Autodesk Inventor part; units mm, degrees
ref_plane "YZ Plane" through (0, 0, 0) normal (1, 0, 0) x (0, 1, 0)
ref_plane "XZ Plane" through (0, 0, 0) normal (0, 1, 0) x (-1, 0, 0)
ref_plane "XY Plane" through (0, 0, 0) normal (0, 0, 1) x (1, 0, 0)
sketch "Sketch1" plane through (0, 0, 0) normal (0, 0, 1) x (1, 0, 0)
  line L0 (0, 0) -> (-25.4, 0)
  line L1 (-25.4, 0) -> (-25.4, 50.8)
  line L2 (-25.4, 50.8) -> (0, 50.8)
  line L3 (0, 50.8) -> (0, 0)
  line L4 (-22.225, 3.175) -> (-3.175, 3.175)
  line L5 (-3.175, 3.175) -> (-3.175, 47.625)
  line L6 (-3.175, 47.625) -> (-22.225, 47.625)
  line L7 (-22.225, 47.625) -> (-22.225, 3.175)
  dimension "d0" = 25.4
  dimension "d1" = 50.8
  dimension "d2" = 3.175
extrude "Extrusion1" add sketch "Sketch1" along normal blind 177.8
sketch "Sketch2" plane through (0, 0, 0) normal (1, 0, 0) x (0, 0, -1)
  circle A0 centre (-152.4, 19.05) radius 14.2875
  circle A1 centre (-25.4, 19.05) radius 14.2875
  circle A2 centre (-88.9, 19.05) radius 14.2875
  line L0 (-177.8, 0) -> (-177.8, 50.8)
  line L1 (0, 50.8) -> (0, 0)
  line L2 (0, 50.8) -> (-177.8, 50.8)
  line L3 (0, 0) -> (-177.8, 0)
  dimension "d5" = 28.575
  dimension "d6" = 28.575
  dimension "d7" = 28.575
  dimension "d8" = 25.4
  dimension "d9" = 25.4
  dimension "d10" = 31.75
  dimension "d11" = 31.75
  dimension "d12" = 19.05
  dimension "a" = 63.5
  dimension "d14" = 63.5
extrude "Extrusion2" cut sketch "Sketch2" against normal blind 209.3722 contours A0 | A1 | A2
properties part number "Clamp Arms"
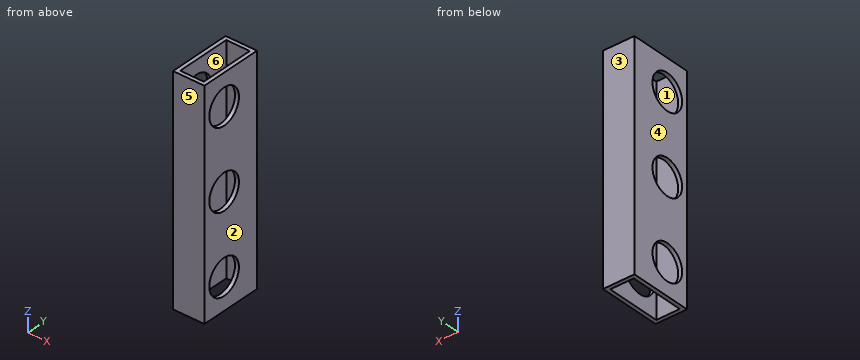
Verification items for the finished model (mm, model axes). Face numbers are marked on the shaded views. A direction names the side the tool comes from. Coordinates: 2 decimals unless noted, no trailing zeros. Order: outer loops, then holes, each group sorted by start corner. A loop starts at its lowest first (then second) coordinate and runs counter-clockwise, first axis right, second up. Notation, with made-up numbers: M 41.25,75.25 L 88.25,75.25 A24 ccw 88.25,107.25 Z; hole C 7.5,29.5 d9. An arc over 180 degrees is marked long. One line per item, written item: value. Start each with the question number.
Item 1: Sectioned sample at C-C on x = -18.75. Record the cut outline in (y, z) (3 decimals).
Item 2: Sectioned sample at A-A on z = 25.4. Record the cut outline in (x, y) (1 decimal), then the cut area to 3 significant figures.
Item 3: Sectioned sample at B-B on y = 19.05. Give the number of separate pieces and of enclosed holes in the cut face, then the cut area to 3 significant figures.
Item 4: Sectioned sample at D-D on z = 43.5. Record the cut outline in (x, y) (3 decimals).
Item 5: Access from +Z, -Z, +X, -X, +Y, -Y to the whole of each face (thin tool, end or side, straight path). Record for the marked faces 1 and 2.
Item 6: Depth check by flat-ended pin: P1, Ø15, axis at x = -14, z = 107, coming from the -Y side. Enter the tip coordinate at first touch or a pass-through.
Item 7: Thickness scan on probe 1 along Y at (x, z) = (-24.2, 152.4); probe 2 along Y at (x, z) = (-12.75, 56) (3 decimals); probe 3 along X at (y, z) = (11, 55) (3 decimals). Record the ranges inside material, lowest first.
Item 8: Mould release check, pull along Y, two halves, no side actions. Record for the marked faces 3, 4, 5 and 6: pulls with the +Y half, pulls with the -Y half, needs draft (parallel to the pull), parting line crosses it, or undercut.
Calculated:
1. outline: M 0,0 L 3.175,0 L 3.175,177.8 L 0,177.8 Z; M 47.625,0 L 50.8,0 L 50.8,177.8 L 47.625,177.8 Z
2. outline: M -25.4,0 L 0,0 L 0,4.8 L -3.2,4.8 L -3.2,3.2 L -22.2,3.2 L -22.2,4.8 L -25.4,4.8 Z; M -25.4,33.3 L -22.2,33.3 L -22.2,47.6 L -3.2,47.6 L -3.2,33.3 L 0,33.3 L 0,50.8 L -25.4,50.8 Z
2. area: 262 mm^2
3. separate pieces: 8
3. enclosed holes: 0
3. area: 585 mm^2
4. outline: M -25.4,0 L 0,0 L 0,50.8 L -25.4,50.8 Z; hole M -22.225,3.175 L -3.175,3.175 L -3.175,47.625 L -22.225,47.625 Z
5. face 1: +Z, -Z
5. face 2: +Z, -Z, +X, +Y, -Y
6. P1: y = 0
7. probe 1: 0 to 4.76, 33.34 to 50.8
7. probe 2: 0 to 3.175, 47.625 to 50.8
7. probe 3: -25.4 to -22.225, -3.175 to 0
8. face 3: pulls with the +Y half
8. face 4: needs draft
8. face 5: pulls with the -Y half
8. face 6: undercut
